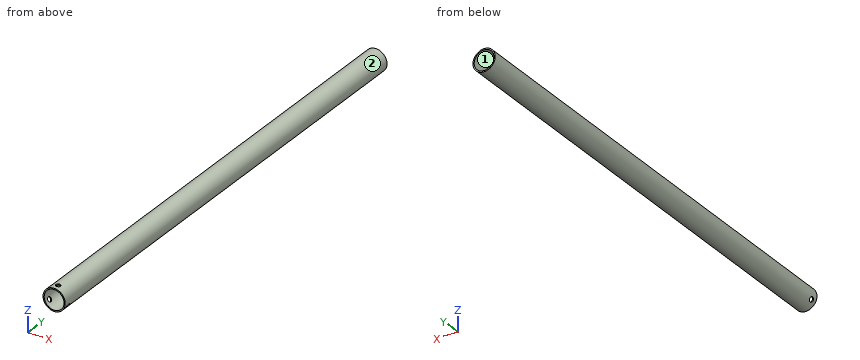
Autodesk Inventor part; units mm, degrees
ref_plane "Plano de trabajo1" through (0, 0, 18.5) normal (0, 0, 1) x (1, 0, 0)
ref_plane "Plano de trabajo2" through (18.5, 0, 0) normal (1, 0, 0) x (0, 1, 0)
ref_plane "XZ Plane" through (0, 0, 0) normal (0, 1, 0) x (-1, 0, 0)
sketch "Boceto1" plane through (0, 0, 0) normal (0, 1, 0) x (-1, 0, 0)
  circle A0 centre (0, 0) radius 18.5
  dimension "d0" = 37
extrude "Extrusión1" add sketch "Boceto1" along normal blind 805
shell "Vaciado1" thickness 2 removed faces 2 at (3.5031, 0, 5.0751) at (3.5031, 805, 5.0751)
ref_plane "Plano de trabajo1" through (0, 0, 18.5) normal (0, 0, 1) x (1, 0, 0)
ref_plane "Plano de trabajo2" through (18.5, 0, 0) normal (1, 0, 0) x (0, 1, 0)
sketch "Boceto4" plane through (0, 0, 18.5) normal (0, 0, 1) x (1, 0, 0)
  line L0 (0, 18.0734) -> (0, -36.4146) construction
  line L1 (47.7272, 0) -> (-52.5468, 0) construction
  circle A0 centre (0, 10) radius 4
  point P0 (0, 0)
  dimension "d14" = 8
  dimension "d15" = 10
extrude "Extrusión4" cut sketch "Boceto4" against normal blind 10
pattern_circular "Patrón circular1" count 3 over 360 about axis through (0, 0, 0) along (0, 1, 0) of "Extrusión4"
The listing builds one solid part. Answer for the finished solid, in the listing's coordinates (mm). Face numbers are marked on the shaded views. Coordinates: 2 decimals unless noted, no trailing zeros. Write each loop counter-clockwise with the first axis right and the second up, starting at its lowest first coordinate (ties: lowest second). Pieces come first, ordered by that corner, then holes. Notation, with made-up numbers: (42, -21) - (61, -21) arc R33 ccw to (61, 18) - close; hole circle Ø9 at (72.25, -7). An arc over 180 degrees is marked (long way). Return JSON: item names as keys, results as strings. Group by question number.
Q1. Flat-ended cylindrical pins translate along their axes: pin 1 Ø1 at (x, y) = (6, 675) entering from -Z; pin 2 Ø1.5 at (x, z) = (15, -14) entering from -Y; pin 3 Ø6 at (y, z) = (521.5, 11) entering from -X; pin 4 Ø1.5 at (y, z) = (272.5, 2) entering from +X. Find the tip coordinate at first contact, or state that the pin passes through.
Q2. The part is cut by section A-A on z = 9. Write down the section's boundary in (x, y), and give its area (3 significant figures).
Q3. For a pull along Z with two mould halves and no side action, classify the marked faces 1 and 2 as +Z half, -Z half, draft (parallel to the pull), parting line (faces both ways), or undercut.
Q4. Find the intervals of material crossed by line 1 along Z through (x, y) = (0, 422); line 2 along Y through (x, z) = (0, 17.9); line 3 along X through (y, z) = (87, 1), in increasing order. Write a range as [from, to].
Q5. The part is cut by section B-B on y = 669. Write down the section's boundary in (x, z).
Evaluation:
{
 "1": {"pin 1": "stops at z = -17.66", "pin 2": "passes through", "pin 3": "stops at x = -16.68", "pin 4": "stops at x = 18.46"},
 "2": {"outline": "(-16.16, 0) - (-13.83, 0) - (-13.83, 805) - (-16.16, 805) - close; (13.83, 0) - (16.16, 0) - (16.16, 805) - (13.83, 805) - close", "area": "3,760 mm2"},
 "3": {"face 1": "undercut", "face 2": "parting line"},
 "4": {"line 1": "z = [-18.5, -16.5], [16.5, 18.5]", "line 2": "y = [0, 6], [14, 805]", "line 3": "x = [-18.47, -16.47], [16.47, 18.47]"},
 "5": {"outline": "circle Ø37 at (0, 0); hole circle Ø33 at (0, 0)"}
}
